Model file for the job. Use its own axes, mm. A direction names the side the tool comes from. Round coordinates to 2 decimals unless told otherwise and drop trailing zeros. Write each loop counter-clockwise with the first axis right and the second up, starting at its lowest first coordinate (ties: lowest second). Pieces come first, ordered by that corner, then holes. Notation, with made-up numbers: (66.25, 18.25) - (86.25, 18.25) arc R19 cw to (86.25, 42.25) - close; hole circle Ø6 at (54, 40.5). An arc over 180 degrees is marked (long way). One line per item, written item: value.
from build123d import *

# Parameters (mm, degrees)
SKETCH2_R          = 11.88832093
CUT_EXTRUDE2_DEPTH = 10
CHAMFER1_SIZE      = 0.5
SKETCH3_R          = 0.1
CUT_EXTRUDE3_DEPTH = 14


with BuildPart() as part:
    # Sketch1 → Revolve1 (revolve)
    with BuildSketch(Plane(origin=(0, 0, 0), x_dir=(1, 0, 0), z_dir=(0, 1, 0))):
        Polygon((1, 8.5), (3, 8.5), (3, 3.5), (4, 3.5), (4, 0), (0.85, -4.5), (0, -4.5), (0, -3.5), (1, -1.767949192), align=None)
    revolve(axis=Axis((0, 0, 0), (0, 0, 1)))

    # Sketch2 → Cut-Extrude2 (cut)
    with BuildSketch(Plane(origin=(0, 0, -3.5), x_dir=(-1, 0, 0), z_dir=(0, 0, -1))):
        Circle(SKETCH2_R)
        Polygon((3.25, 1.876388375), (0, 3.75277675), (-3.25, 1.876388375), (-3.25, -1.876388375), (0, -3.75277675), (3.25, -1.876388375), align=None, mode=Mode.SUBTRACT)
    extrude(amount=-CUT_EXTRUDE2_DEPTH, mode=Mode.SUBTRACT)

    # Chamfer1
    chamfer1_edges = [part.edges().sort_by_distance(p)[0] for p in [
        (-3, 0, -8.5),
    ]]
    chamfer(chamfer1_edges, length=CHAMFER1_SIZE)

    # Sketch3 → Cut-Extrude3 (cut, through all)
    with BuildSketch(Plane.XY.offset(4.5)):
        Circle(SKETCH3_R)
    extrude(amount=-CUT_EXTRUDE3_DEPTH, mode=Mode.SUBTRACT)


solid = part.part
1. Mould opens along X. For faces 3 (the face through (-3, 0, -6)), 4 (the face through (1, -3, -3.5)), 5 (the face through (0.435, 0.137, 2.71)) say: released by +X, released by -X, zero draft, split by the parting line, or undercut.
Report:
face 3: split by the parting line
face 4: zero draft
face 5: undercut
2. Band-saw the part on B-B on z = -7.25. Write the cut outline in (x, y), plus the area to 3 significant figures.
Report:
outline: circle Ø6 at (0, 0); hole circle Ø2 at (0, 0)
area: 25.1 mm²
3. Wall check: probe 1 along Y at (x, z) = (-0.5, -1.75); probe 2 along Z at (x, y) = (-1, 2.5); probe 3 along Z at (x, y) = (-1.5, -1.25). Give the ranges that are in metal, low to high. Write a range as [from, to].
Report:
probe 1: [-3.46, -0.87], [0.87, 3.46]
probe 2: [-8.31, 1.87]
probe 3: [-8.5, 2.92]
4. Band-saw the part on A-A on z = -1.25. Write the cut outline in (x, y).
Report:
outline: (-3.25, -1.88) - (0, -3.75) - (3.25, -1.88) - (3.25, 1.88) - (0, 3.75) - (-3.25, 1.88) - close; hole circle Ø2 at (0, 0)
5. Tool access for faces 1 (the face through (0, -1, -3)), 2 (the face through (-1.65, 2.8, -1.25)): list every direction of +Z, -Z, +X, -X, +Y, -Y with a clear straight run to the whole face (end or side of a thin tool).
Report:
face 1: -Z
face 2: +Z, -Z, -X, +Y
6. Drop flat-ended pins along their axis: pin 1 (1.5 mm diameter, centred on x = -0.5, z = -5.5, fed in from +Y); pin 2 (4 mm diameter, centred on y = 2.5, z = -5.5, fed in from +X). Give the stop position or say it passes through.
Report:
pin 1: y = 3
pin 2: x = 2.96
